CAD build for the part. Positions are in the model's coordinates, mm. Coordinates: 2 decimals unless noted, no trailing zeros. Write each loop counter-clockwise with the first axis right and the second up, starting at its lowest first coordinate (ties: lowest second). Pieces come first, ordered by that corner, then holes.
Autodesk Inventor part; units mm, degrees
ref_plane "YZ Plane" through (0, 0, 0) normal (1, 0, 0) x (0, 1, 0)
ref_plane "XZ Plane" through (0, 0, 0) normal (0, 1, 0) x (-1, 0, 0)
ref_plane "XY Plane" through (0, 0, 0) normal (0, 0, 1) x (1, 0, 0)
sketch "Sketch1" plane through (0, 0, 0) normal (0, 0, 1) x (1, 0, 0)
  line L0 (-520.7, -1549.4) -> (520.7, -1549.4)
  line L1 (520.7, -1549.4) -> (520.7, 1549.4)
  line L2 (520.7, 1549.4) -> (-520.7, 1549.4)
  line L3 (-520.7, 1549.4) -> (-520.7, -1549.4)
  line L4 (-520.7, -1549.4) -> (520.7, 1549.4) construction
  line L5 (520.7, -1549.4) -> (-520.7, 1549.4) construction
  line L6 (-520.7, 0) -> (520.7, 0)
  line L7 (520.7, 0) -> (-520.7, -1549.4)
  line L8 (-483.8087, -1574.1958) -> (-557.5913, -1524.6042)
  line L9 (557.5913, -24.7958) -> (483.8087, 24.7958)
  line L10 (483.8087, 24.7958) -> (-557.5913, -1524.6042)
  line L11 (-483.8087, -1574.1958) -> (557.5913, -24.7958)
  line L12 (483.8087, 24.7958) -> (520.7, 79.6829)
  line L13 (-520.7, 1549.4) -> (520.7, -1549.4) construction
  line L14 (520.7, 0) -> (-520.7, 1549.4)
  line L15 (-483.8087, 1574.1958) -> (-557.5913, 1524.6042)
  line L16 (557.5913, 24.7958) -> (483.8087, -24.7958)
  line L17 (483.8087, -24.7958) -> (-557.5913, 1524.6042)
  line L18 (-483.8087, 1574.1958) -> (557.5913, 24.7958)
  line L19 (483.8087, -24.7958) -> (520.7, -79.6829)
  point P0 (0, 0)
  point P1 (520.7, 79.6829)
  point P2 (-467.1426, 1549.4)
  point P3 (-520.7, 1469.7171)
  point P4 (520.7, -79.6829)
  point P5 (520.7, -79.6829)
  point P6 (467.1426, 0)
  point P7 (-520.7, -1469.7171)
  point P8 (-467.1426, -1549.4)
  dimension "d0" = 1041.4
  dimension "d1" = 3098.8
  dimension "d3" = 88.9
  dimension "d4" = 88.9
extrude "Extrusion1" add sketch "Sketch1" along normal blind 38.1 contours L7 L19 L11 L0 | L3 L10 L17 L19 L7
properties part number "S_2x4x73.498"
Item 1: Flat gauge pins, fed straight in: pin 1 Ø8 at (y, z) = (-781.5, 5) entering from +X; pin 2 Ø1.5 at (y, z) = (-371, 18) entering from -X; pin 3 Ø5 at (x, z) = (-324.5, 13) entering from +Y. Where does each tip first touch, or does it go through?
Item 2: Saw through at A-A, the plane z = 8.5. Write the cut outline in (x, y), and give its area (3 significant figures).
Item 3: Saw through at B-B, the plane x = 195.5. Write the cut outline in (y, z), and give its area (3 significant figures).
Item 4: Saw through at C-C, the plane y = -370. Write the cut outline in (x, z).
Item 5: Wall check: line 1 along Y through (x, z) = (-116, 4); line 2 along X through (y, z) = (-757, 11); line 3 along X through (y, z) = (-1069.5, 30.5). Give the ranges that are in metal, low to high.
Working result:
1. pin 1: stops at x = 51.68
1. pin 2: stops at x = 217.28
1. pin 3: stops at y = -1174.09
2. outline: (-520.7, -1549.4) - (-467.14, -1549.4) - (520.7, -79.68) - (483.81, -24.8) - (467.14, 0) - (-520.7, -1469.72) - close
2. area: 160,000 mm2
3. outline: (-563.52, 0) - (-404.15, 0) - (-404.15, 38.1) - (-563.52, 38.1) - close
3. area: 6,070 mm2
4. outline: (218.45, 0) - (325.57, 0) - (325.57, 38.1) - (218.45, 38.1) - close
5. line 1: y = -1026.97 to -867.6
5. line 2: x = -41.66 to 65.45
5. line 3: x = -251.7 to -144.59
